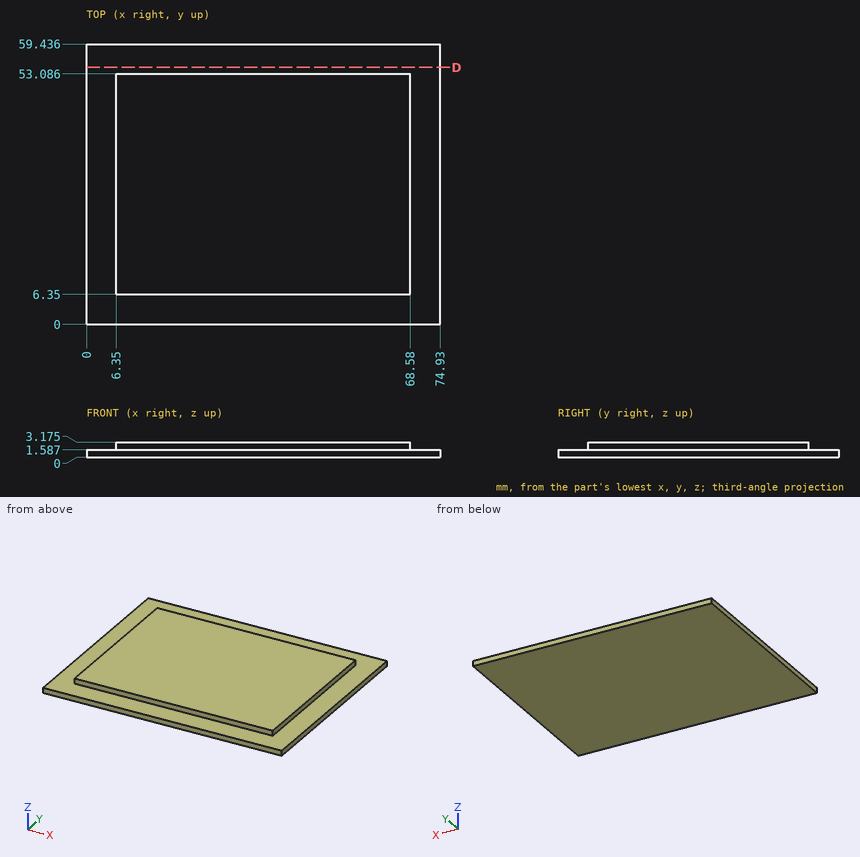
Study the drawing (mm; zero at the part's minimum x, y, z) and answer. Give positions to 0.01 mm unless a question says otherwise; leave off trailing zeros. Write each loop counter-clockwise with the first axis right and the second up, starting at its lowest first coordinate (ties: lowest second). Pieces come first, ordered by that corner, then holes. Notation, with made-up numbers: M 11,49 L 63,49 A16 cw 63,64 Z; hole C 76.25,23.5 d5. An arc over 180 degrees is marked long. Put each result on its own line as item: value. Start each with the question number.
1. Consider line 1 along X through (y, z) = (26, 2.75); line 2 along Z through (x, y) = (66.5, 57.5). Determine where each line is inside the solid, lowest interval first.
2. The part is cut by section D-D, the plane y = 54.5. Give the vertices of the cut face in (x, z), and give its area (3 significant figures).
3. Each of these flat-tipped pins is pushed along its axis until it touches: pin 1 Ø0.8 at (y, z) = (19.5, 3) entering from +X; pin 2 Ø1.7 at (x, z) = (47, 2.5) entering from +Y; pin 3 Ø1.3 at (x, z) = (29, 2.5) entering from -Y. Where does it stop, or does it pass through?
Final values:
1. line 1: x = 6.35 to 68.58
1. line 2: z = 0 to 1.59
2. outline: M 0,0 L 74.93,0 L 74.93,1.59 L 0,1.59 Z
2. area: 119 mm²
3. pin 1: stops at x = 68.58
3. pin 2: stops at y = 53.09
3. pin 3: stops at y = 6.35
